Source: CAD feature listing. Evaluate the final solid. Frame: model axes, mm. A direction names the side the tool comes from. Coordinates: 2 decimals unless noted, no trailing zeros. Loops run counter-clockwise (first coordinate to the right, second up) from the corner with the lowest first, then second, coordinate; pieces in that order, holes last. Notation, with made-up numbers: M 60,85.25 L 119,85.25 A22 cw 119,118.25 Z; hole C 3.25,79.5 d8. An arc over 180 degrees is marked long. Write each question's results on one line, items separated by ' | '. Start each with the question number.
Autodesk Inventor part; units mm, degrees
ref_plane "YZ Plane" through (0, 0, 0) normal (1, 0, 0) x (0, 1, 0)
ref_plane "XZ Plane" through (0, 0, 0) normal (0, 1, 0) x (-1, 0, 0)
ref_plane "XY Plane" through (0, 0, 0) normal (0, 0, 1) x (1, 0, 0)
sketch "Sketch1" plane through (0, 0, 0) normal (0, 0, 1) x (1, 0, 0)
  line L0 (-34.86, 0) -> (34.86, 0) construction
  line L1 (0, -34.86) -> (0, 34.86) construction
  line L2 (0, 0) -> (11.1575, 11.1575) construction
  line L3 (0, 0) -> (15.7791, 0) construction
  line L4 (0, 24.9) -> (16.8009, 24.9)
  line L5 (16.8009, 24.9) -> (16.8009, 21.2415)
  line L6 (16.8009, 21.2415) -> (19.0212, 19.0212)
  line L7 (24.9, 0) -> (24.9, 16.8009)
  line L8 (24.9, 16.8009) -> (21.2415, 16.8009)
  line L9 (21.2415, 16.8009) -> (19.0212, 19.0212)
  line L10 (0, -24.9) -> (16.8009, -24.9)
  line L11 (16.8009, -24.9) -> (16.8009, -21.2415)
  line L12 (16.8009, -21.2415) -> (19.0212, -19.0212)
  line L13 (24.9, 0) -> (24.9, -16.8009)
  line L14 (24.9, -16.8009) -> (21.2415, -16.8009)
  line L15 (21.2415, -16.8009) -> (19.0212, -19.0212)
  line L16 (0, 24.9) -> (-16.8009, 24.9)
  line L17 (-16.8009, 24.9) -> (-16.8009, 21.2415)
  line L18 (-16.8009, 21.2415) -> (-19.0212, 19.0212)
  line L19 (-24.9, 16.8009) -> (-21.2415, 16.8009)
  line L20 (-21.2415, 16.8009) -> (-19.0212, 19.0212)
  line L21 (0, -24.9) -> (-16.8009, -24.9)
  line L22 (-16.8009, -24.9) -> (-16.8009, -21.2415)
  line L23 (-16.8009, -21.2415) -> (-19.0212, -19.0212)
  line L24 (-21.2415, -16.8009) -> (-19.0212, -19.0212)
  line L25 (-24.9, -16.8009) -> (-21.2415, -16.8009)
  line L26 (-24.9, 0) -> (-24.9, -16.8009)
  line L27 (-24.9, 0) -> (-24.9, 16.8009)
  circle A0 centre (0, 0) radius 12.5
  dimension "d0" = 45
  dimension "d2" = 24.9
  dimension "d3" = 3.14
  dimension "d4" = 26.9
  dimension "d5" = 25
extrude "Extrusion1" add sketch "Sketch1" along normal blind 5
sketch "Sketch2" plane through (0, 0, 5) normal (0, 0, 1) x (1, 0, 0)
  circle A0 centre (0, 0) radius 12.5
  line L0 (16.8009, 24.9) -> (-16.8009, 24.9)
  line L1 (-16.8009, 24.9) -> (-16.8009, 21.2415)
  line L2 (-16.8009, 21.2415) -> (-21.2415, 16.8009)
  line L3 (-21.2415, 16.8009) -> (-24.9, 16.8009)
  line L4 (-24.9, 16.8009) -> (-24.9, -16.8009)
  line L5 (-24.9, -16.8009) -> (-21.2415, -16.8009)
  line L6 (-21.2415, -16.8009) -> (-16.8009, -21.2415)
  line L7 (-16.8009, -21.2415) -> (-16.8009, -24.9)
  line L8 (-16.8009, -24.9) -> (16.8009, -24.9)
  line L9 (16.8009, -24.9) -> (16.8009, -21.2415)
  line L10 (16.8009, -21.2415) -> (21.2415, -16.8009)
  line L11 (21.2415, -16.8009) -> (24.9, -16.8009)
  line L12 (24.9, -16.8009) -> (24.9, 16.8009)
  line L13 (24.9, 16.8009) -> (21.2415, 16.8009)
  line L14 (21.2415, 16.8009) -> (16.8009, 21.2415)
  line L15 (16.8009, 21.2415) -> (16.8009, 24.9)
  line L16 (-34.86, 0) -> (34.86, 0) construction
  line L17 (0, -34.86) -> (0, 34.86) construction
  line L18 (-10, 23.4) -> (10, 23.4)
  line L19 (10, 23.4) -> (10, 20.4)
  line L20 (10, 20.4) -> (-10, 20.4)
  line L21 (-10, 20.4) -> (-10, 23.4)
  line L22 (-10, -23.4) -> (10, -23.4)
  line L23 (10, -23.4) -> (10, -20.4)
  line L24 (10, -20.4) -> (-10, -20.4)
  line L25 (-10, -20.4) -> (-10, -23.4)
  dimension "d8" = 20
  dimension "d9" = 3
  dimension "d10" = 1.5
  dimension "d19" = 40.8
  dimension "d20" = 46.8
extrude "Extrusion2" add sketch "Sketch2" along normal blind 7 contours L18 L19 L20 L21 | L25 L24 L23 L22
chamfer "Fase1" distance 0.7 distance2 7 1 edges at (0, 23.4, 12) measured on face at (3.3333, 21.4, 12)
chamfer "Fase2" distance 0.7 distance2 7 1 edges at (0, -23.4, 12) measured on face at (-3.3333, -21.4, 12)
properties part number "20_Cube_insert_Sample_holder"
Item 1: Line query: probe 1 along Y at (x, z) = (0, 1.95); probe 2 along Z at (x, y) = (13.5, -22); probe 3 along Y at (x, z) = (22.5, 2.75). Output: solid intervals per line, ascending.
Item 2: Cut plane A-A (y = 0). Output: boundary loops of the cut face in (x, z).
Item 3: Cut plane C-C (z = 2). Output: boundary loops of the cut face in (x, y).
Item 4: Cut plane D-D (z = 9). Output: boundary loops of the cut face in (x, y).
Item 5: First-contact query: pin 1 Ø2.5 at (y, z) = (-22.5, 8.5) entering from -X; pin 2 Ø1.5 at (y, z) = (21.5, 7.5) entering from +X; pin 3 Ø15 at (x, y) = (0, 0) entering from -Z (3 decimals); pin 4 Ø1 at (x, z) = (-4.5, 6) entering from -Y. Flat tips, straight axial feed; report the tip coordinate or a pass-through.
Item 6: Mould query, pull axis Y, two halves, no side actions, for faces 4 (the flat face through (-19.05, 18.99, 2.46)), 5 (the flat face through (23, -16.801, 2)), 6 (the flat face through (-11.4, 5.9, 5)), 7 (the flat face through (-16.801, 23, 2)). Classes: +Y half, -Y half, draft (parallel to the pull), parting line (faces both ways), or undercut.
Item 7: Access query for faces 1 (the flat face through (23, 16.801, 2)), 2 (the flat face through (-10, 22, 8)), 3 (the flat face through (10, -22, 8)). Directions: +Z, -Z, +X, -X, +Y, -Y. A direction counts if a zero-diameter tool reaches every point of the face in a straight line with its end or side. Return the directions, or none.
Response values:
1) probe 1: y = -24.9 to -12.5, 12.5 to 24.9 | probe 2: z = 0 to 5 | probe 3: y = -16.8 to 16.8
2) outline: M -24.9,0 L -12.5,0 L -12.5,5 L -24.9,5 Z; M 12.5,0 L 24.9,0 L 24.9,5 L 12.5,5 Z
3) outline: M -24.9,-16.8 L -21.24,-16.8 L -16.8,-21.24 L -16.8,-24.9 L 16.8,-24.9 L 16.8,-21.24 L 21.24,-16.8 L 24.9,-16.8 L 24.9,16.8 L 21.24,16.8 L 16.8,21.24 L 16.8,24.9 L -16.8,24.9 L -16.8,21.24 L -21.24,16.8 L -24.9,16.8 Z; hole C 0,0 d25
4) outline: M -10,-23 L 10,-23 L 10,-20.4 L -10,-20.4 Z; M -10,20.4 L 10,20.4 L 10,23 L -10,23 Z
5) pin 1: stops at x = -10 | pin 2: stops at x = 10 | pin 3: passes through | pin 4: stops at y = -23.35
6) face 4: +Y half | face 5: -Y half | face 6: undercut | face 7: draft
7) face 1: +Z, -Z, +X, +Y | face 2: +Z, -X, +Y, -Y | face 3: +Z, +X, +Y, -Y
